from build123d import *

# Parameters (mm, degrees)
SKETCH_1_W           = 400
SKETCH_1_H           = 329
EXTRUDE_1_DEPTH      = 25
SKETCH_2_W           = 400
SKETCH_2_H           = 162
EXTRUDE_2_DEPTH      = 27
SKETCH_4_W           = 400
SKETCH_4_H           = 9
SKETCH_4_H_2         = 13
EXTRUDE_3_DEPTH      = 9
CUT_EXTRUDE_3_DEPTH  = 400
SKETCH_10_R          = 2
CUT_EXTRUDE_8_DEPTH  = 9.03
EXTRUDE_START        = 0.07
SKETCH_12_W          = 14.540639504
SKETCH_12_H          = 329
SKETCH_12_R          = 2
EXTRUDE_4_DEPTH      = 0.07
EXTRUDE_5_DEPTH      = 329
SKETCH_15_R          = 3.5
CUT_EXTRUDE_10_DEPTH = 22


with BuildPart() as part:
    # 草图1 → 凸台-拉伸1 (new body)
    with BuildSketch(Plane(origin=(0, 0, 0), x_dir=(1, 0, 0), z_dir=(0, 1, 0))):
        with Locations((200, 164.5)):
            Rectangle(SKETCH_1_W, SKETCH_1_H)
    extrude(amount=EXTRUDE_1_DEPTH)

    # 草图2 → 凸台-拉伸2 (add)
    with BuildSketch(Plane(origin=(0, 25, 0), x_dir=(1, 0, 0), z_dir=(0, 1, 0))):
        with Locations((200, 168)):
            Rectangle(SKETCH_2_W, SKETCH_2_H)
    extrude(amount=EXTRUDE_2_DEPTH)

    # 草图4 → 凸台-拉伸3 (add)
    with BuildSketch(Plane(origin=(0, 25, 0), x_dir=(1, 0, 0), z_dir=(0, 1, 0))):
        with Locations((200, 324.5)):
            Rectangle(SKETCH_4_W, SKETCH_4_H)
        with Locations((200, 6.5)):
            Rectangle(SKETCH_4_W, SKETCH_4_H_2)
    extrude(amount=EXTRUDE_3_DEPTH)

    # 草图8 → 切除-拉伸3 (cut)
    with BuildSketch(Plane(origin=(0, 0, -329), x_dir=(-1, 0, 0), z_dir=(0, 0, -1))):
        Polygon((-267.5, 5), (-267.5, 0), (-114.958104289, 0), (-118.459360496, 13.066866054), (-133, 13.066866054), (-133, 5), align=None)
    extrude(amount=-CUT_EXTRUDE_3_DEPTH, mode=Mode.SUBTRACT)

    # 草图10 → 切除-拉伸8 (cut)
    with BuildSketch(Plane.XZ.offset(-13.066866054)):
        with Locations(Location((124.5, -37, 0), (0, 0, 270))):
            Circle(SKETCH_10_R)
        with Locations(Location((124.5, -63, 0), (0, 0, 270))):
            Circle(SKETCH_10_R)
        with Locations(Location((124.5, -89, 0), (0, 0, 270))):
            Circle(SKETCH_10_R)
        with Locations(Location((124.5, -115, 0), (0, 0, 270))):
            Circle(SKETCH_10_R)
        with Locations(Location((124.5, -141, 0), (0, 0, 270))):
            Circle(SKETCH_10_R)
        with Locations(Location((124.5, -167, 0), (0, 0, 270))):
            Circle(SKETCH_10_R)
        with Locations(Location((124.5, -193, 0), (0, 0, 270))):
            Circle(SKETCH_10_R)
        with Locations(Location((124.5, -219, 0), (0, 0, 270))):
            Circle(SKETCH_10_R)
        with Locations(Location((124.5, -245, 0), (0, 0, 270))):
            Circle(SKETCH_10_R)
    extrude(amount=-CUT_EXTRUDE_8_DEPTH, mode=Mode.SUBTRACT)

    # 草图12 → 凸台-拉伸4 (add)
    with BuildSketch(Plane.XZ.offset(-13.066866054).offset(EXTRUDE_START)):
        with Locations((125.729680248, -164.5)):
            Rectangle(SKETCH_12_W, SKETCH_12_H)
        with Locations(Location((124.5, -63, 0), (0, 0, 270))):
            Circle(SKETCH_12_R, mode=Mode.SUBTRACT)
        with Locations(Location((124.5, -115, 0), (0, 0, 270))):
            Circle(SKETCH_12_R, mode=Mode.SUBTRACT)
        with Locations(Location((124.5, -167, 0), (0, 0, 270))):
            Circle(SKETCH_12_R, mode=Mode.SUBTRACT)
        with Locations(Location((124.5, -219, 0), (0, 0, 270))):
            Circle(SKETCH_12_R, mode=Mode.SUBTRACT)
        with Locations(Location((124.5, -245, 0), (0, 0, 270))):
            Circle(SKETCH_12_R, mode=Mode.SUBTRACT)
        with Locations(Location((124.5, -193, 0), (0, 0, 270))):
            Circle(SKETCH_12_R, mode=Mode.SUBTRACT)
        with Locations(Location((124.5, -141, 0), (0, 0, 270))):
            Circle(SKETCH_12_R, mode=Mode.SUBTRACT)
        with Locations(Location((124.5, -89, 0), (0, 0, 270))):
            Circle(SKETCH_12_R, mode=Mode.SUBTRACT)
        with Locations(Location((124.5, -37, 0), (0, 0, 270))):
            Circle(SKETCH_12_R, mode=Mode.SUBTRACT)
    extrude(amount=-EXTRUDE_4_DEPTH)

    # 草图13 → 凸台-拉伸5 (add)
    with BuildSketch(Plane.XY):
        Polygon((118.459360496, 13.066866054), (118.459360496, 12.996866054), (118.440604053, 12.996866054), align=None)
    extrude(amount=-EXTRUDE_5_DEPTH)

    # 草图15 → 切除-拉伸10 (cut)
    with BuildSketch(Plane(origin=(400, 0, 0), x_dir=(0, 0, -1), z_dir=(1, 0, 0))):
        with Locations((207, 39.026793109)):
            Circle(SKETCH_15_R)
        with Locations((207, 7.026793109)):
            Circle(SKETCH_15_R)
        with Locations((167, 39.026793109)):
            Circle(SKETCH_15_R)
        with Locations((167, 7.026793109)):
            Circle(SKETCH_15_R)
        with Locations((127, 39.026793109)):
            Circle(SKETCH_15_R)
        with Locations((127, 7.026793109)):
            Circle(SKETCH_15_R)
    extrude(amount=-CUT_EXTRUDE_10_DEPTH, mode=Mode.SUBTRACT)


solid = part.part
Can you work these out from the model? Positions are in its coordinate system, mm. A direction names the side the tool comes from. Give positions to 0.01 mm unless a question says otherwise; leave off trailing zeros. Loops run counter-clockwise (first coordinate to the right, second up) from the corner with the lowest first, then second, coordinate; pieces in that order, holes last. Notation, with made-up numbers: M 51,31 L 68,31 A22 cw 68,60 Z; hole C 77.5,3 d9. An arc over 180 degrees is marked long. One line per item, written item: value. Start each with the question number.
1) If we section it at C-C, the plane x = 147.5: Write out the boundary of the cut face in (y, z).
2) If we section it at A-A, the plane x = 56: Write out the boundary of the cut face in (y, z), and give its area (3 significant figures).
3) Thinking about a two-plate mould opening in X: for faces 4 (the face through (126, 12.997, -162)), 5 (the face through (400, 20, -162)), 6 (the face through (197, 34, -7)), 7 (the face through (116.675, 6.407, -166.803)), which applies, +X half, -X half, draft (parallel to the pull), parting line (faces both ways), or undercut?
4) I'm going to push flat-ended pins straight in: pin 1 (4.5 mm diameter, centred on x = 124, z = -37.5, fed in from -Y); pin 2 (1.2 mm diameter, centred on x = 125, z = -167.5, fed in from -Y); pin 3 (11 mm diameter, centred on y = 7.03, z = -167, fed in from +X); pin 4 (3.5 mm diameter, centred on y = 8, z = -206.5, fed in from +X). Where does each tip first touch, or does it pass through?
5) If we section it at B-B, the plane z = -274.5: Write out the boundary of the cut face in (x, y), and give its area (3 significant figures).
6) If I drill on line 1 (Y direction, x = 384, z = -127); line 2 (Z direction, x = 73, y = 26.5); line 3 (X direction, y = 16, z = -167), over which ranges is the centre line in solid material (lowest first)? Write a range as [from, to].
7) On a 3-axis mill with a long thin cutter (end or side, diameter ignored), from which of +Z, -Z, +X, -X, +Y, -Y can I reach the whole of each face in a straight line? I mean faces 1 (the face through (133, 9, -167)), 2 (the face through (203, 17, 0)), 3 (the face through (197, 38, -87)). Say none if no direction works.
Completed:
1. outline: M 5,-329 L 34,-329 L 34,-320 L 25,-320 L 25,-249 L 52,-249 L 52,-87 L 25,-87 L 25,-13 L 34,-13 L 34,0 L 5,0 Z
2. outline: M 0,-329 L 34,-329 L 34,-320 L 25,-320 L 25,-249 L 52,-249 L 52,-87 L 25,-87 L 25,-13 L 34,-13 L 34,0 L 0,0 Z
2. area: 12,800 mm^2
3. face 4: undercut
3. face 5: +X half
3. face 6: draft
3. face 7: undercut
4. pin 1: stops at y = 13
4. pin 2: stops at y = 22.1
4. pin 3: stops at x = 400
4. pin 4: stops at x = 378
5. outline: M 0,0 L 114.96,0 L 118.44,13 L 133,13 L 133,5 L 267.5,5 L 267.5,0 L 400,0 L 400,25 L 0,25 Z
5. area: 9,120 mm^2
6. line 1: y = [0, 3.53], [10.53, 35.53], [42.53, 52]
6. line 2: z = [-329, -320], [-249, -87], [-13, 0]
6. line 3: x = [0, 122.5], [126.5, 400]
7. face 1: +Z, -Z, -Y
7. face 2: +Z, +X, -X, +Y, -Y
7. face 3: +X, -X, +Y
